For this review, use the dimensioned drawing (mm, ordinates from the lowest corner) and the shaded views. Coordinates: 2 decimals unless noted, no trailing zeros. Write each loop counter-clockwise with the first axis right and the second up, starting at its lowest first coordinate (ties: lowest second). Pieces come first, ordered by that corner, then holes. Notation, with made-up numbers: (53, 5.5) -> (107, 5.5) arc R34 ccw to (107, 44.5) -> close; hole circle Ø2 at (87.5, 37.25). An arc over 180 degrees is marked (long way). Put each result on its own line as item: value. Start each with the question number.
Item 1: To check wall thickness, follow L1, parallel to X at y = 220.5, z = 10.25; L2, parallel to Y at x = 159, z = 1.5; L3, parallel to Y at x = 183.5, z = 9 (1 decimal). State the ranges of each line that lie inside material, in increasing order.
Item 2: Consider section B-B on y = 109.5. Give the boundary of the cut face in (x, z).
Item 3: Consider section C-C on x = 161. Give the boundary of the cut face in (y, z), and give its area (3 significant figures).
Item 4: Consider section A-A on z = 3.5. Give the boundary of the cut face in (x, y) (1 decimal).
Item 5: Insertion check: P1, Ø1.5, axis at y = 331.5, z = 8, coming from the +X side. The pin has a flat end and moves straight along its axis. Give the tip position at first contact, or say it passes through.
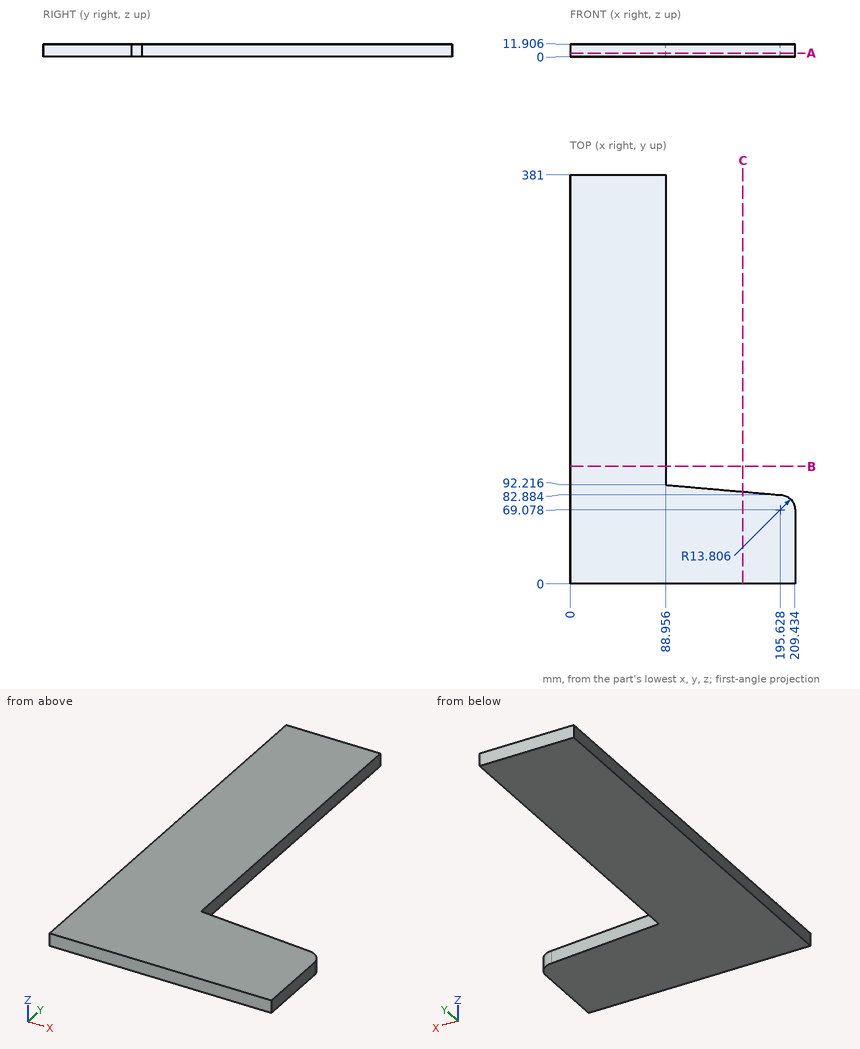
Return value:
1. L1: 0 to 88.96
1. L2: 0 to 86.09
1. L3: 0 to 83.9
2. outline: (0, 0) -> (88.96, 0) -> (88.96, 11.91) -> (0, 11.91) -> close
3. outline: (0, 0) -> (85.91, 0) -> (85.91, 11.91) -> (0, 11.91) -> close
3. area: 1,020 mm^2
4. outline: (0, 0) -> (209.4, 0) -> (209.4, 69.1) arc R13.8 ccw to (195.6, 82.9) -> (89, 92.2) -> (89, 381) -> (0, 381) -> close
5. P1: x = 88.96
